from build123d import *

# Parameters (mm, degrees)
SKETCH1_W                = 21
SKETCH1_H                = 145.5
SKETCH1_W_2              = 11
SKETCH1_H_2              = 21
BOSS_EXTRUDE1_DEPTH      = 2
BOSS_EXTRUDE2_DEPTH      = 30
BOSS_EXTRUDE2_DEPTH_BACK = 2
FILLET2_R                = 2.5
SKETCH6_R                = 2
CUT_EXTRUDE1_DEPTH       = 2
BOSS_EXTRUDE5_DEPTH      = 1
BOSS_EXTRUDE6_DEPTH      = 1
SKETCH9_R                = 2
CUT_EXTRUDE2_DEPTH       = 2
FILLET3_R                = 1


with BuildPart() as part:
    # Sketch1 → Boss-Extrude1 (new body)
    with BuildSketch(Plane.XY):
        Rectangle(SKETCH1_W, SKETCH1_H)
        with Locations((0, -42.75)):
            Rectangle(SKETCH1_W_2, SKETCH1_H_2, mode=Mode.SUBTRACT)
        with Locations((0, 7.25)):
            Rectangle(SKETCH1_W_2, SKETCH1_H_2, mode=Mode.SUBTRACT)
        with Locations((0, 57.25)):
            Rectangle(SKETCH1_W_2, SKETCH1_H_2, mode=Mode.SUBTRACT)
    extrude(amount=BOSS_EXTRUDE1_DEPTH)

    # Sketch2 → Boss-Extrude2 (add, two sides: drawn at the far end of the back side and taken through both)
    with BuildSketch(Plane(origin=(0, 0, 0), x_dir=(-1, 0, 0), z_dir=(0, 0, -1)).offset(-BOSS_EXTRUDE2_DEPTH_BACK)):
        Polygon((10.5, -72.75), (16.5, -72.75), (16.5, -74.75), (-16.5, -74.75), (-16.5, -72.75), align=None)
    extrude(amount=BOSS_EXTRUDE2_DEPTH + BOSS_EXTRUDE2_DEPTH_BACK)

    # Fillet2
    # the kernel refuses this fillet: 2.5 mm, written as the material it takes off along each edge
    with BuildSketch(Plane(origin=(22.623724357, -72.75, -30), x_dir=(0, 0, 1), z_dir=(-1, 0, 0))) as fillet2_piece_1:
        with BuildLine():
            CenterArc((2.449489743, -2.5), FILLET2_R, 90, 78.463040967)
            Line((0, -2), (-0.048989795, -1.99))
            ThreePointArc((-0.048989795, -1.99), (-0.05, -1), (-0.05, 0))
            Line((-0.05, 0), (0, 0.05))
            Line((0, 0.05), (2.449489743, 0.05))
            Line((2.449489743, 0.05), (2.449489743, 0))
        make_face()
    extrude(amount=45.247448714, mode=Mode.SUBTRACT)

    # Sketch6 → Cut-Extrude1 (cut)
    with BuildSketch(Plane(origin=(0, -72.75, 0), x_dir=(1, 0, 0), z_dir=(0, 1, 0))):
        with Locations(Location((0, 24, 0), (0, 0, 270))):
            Circle(SKETCH6_R)
    extrude(amount=-CUT_EXTRUDE1_DEPTH, mode=Mode.SUBTRACT)

    # Sketch7 → Boss-Extrude5 (add, symmetric)
    with BuildSketch(Plane(origin=(7.5, 0, 0), x_dir=(0, 0, -1), z_dir=(1, 0, 0))):
        Polygon((0, -53.25), (12, -72.75), (0, -72.75), align=None)
    extrude(amount=BOSS_EXTRUDE5_DEPTH, both=True)

    # Sketch8 → Boss-Extrude6 (add, symmetric)
    with BuildSketch(Plane(origin=(-7.5, 0, 0), x_dir=(0, 0, -1), z_dir=(1, 0, 0))):
        Polygon((12, -72.75), (0, -53.25), (0, -72.75), align=None)
    extrude(amount=BOSS_EXTRUDE6_DEPTH, both=True)

    # Sketch9 → Cut-Extrude2 (cut)
    with BuildSketch(Plane.XZ.offset(74.75)):
        with Locations(Location((13, -24, 0), (0, 0, 270))):
            Circle(SKETCH9_R)
        with Locations(Location((-13, -24, 0), (0, 0, 90))):
            Circle(SKETCH9_R)
    extrude(amount=-CUT_EXTRUDE2_DEPTH, mode=Mode.SUBTRACT)

    # Fillet3
    fillet3_edges = [part.edges().sort_by_distance(p)[0] for p in [
        (-9.5, -72.75, 0),
        (10.5, -72.75, 1),
        (-10.5, -72.75, 1),
        (9.5, -72.75, 0),
        (6.5, -72.75, -6),
        (8.5, -72.75, -6),
        (0, -72.75, 0),
        (-8.5, -72.75, -6),
        (-6.5, -72.75, -6),
    ]]
    fillet(fillet3_edges, radius=FILLET3_R)


solid = part.part
The model under review builds one solid part; all positions refer to its coordinate system, in mm. A direction names the side the tool comes from. Coordinates: 2 decimals unless noted, no trailing zeros. Loops run counter-clockwise (first coordinate to the right, second up) from the corner with the lowest first, then second, coordinate; pieces in that order, holes last.
(1) Draft analysis for pull direction Z (two halves, no side actions). For faces 1 (the flat face through (8, -63, -6)), 2 (the cylindrical face through (-14.352, -73.764, -25.474)), 3 (the flat face through (0, -6, 2)), 4 (the flat face through (6.5, -66, -3)), state which applies: +Z half, -Z half, draft (parallel to the pull), parting line (faces both ways), or undercut.
Determined:
face 1: -Z half
face 2: undercut
face 3: +Z half
face 4: draft
(2) Consider section D-D, the plane x = 0. Give the boundary of the cut face in (y, z).
Determined:
outline: (-74.75, -30) arc R2.5 ccw to (-72.75, -27.55) - (-72.75, -26) - (-74.75, -26) - close; (-74.75, -22) - (-72.75, -22) - (-72.75, -1) arc R1 cw to (-71.75, 0) - (-53.25, 0) - (-53.25, 2) - (-74.75, 2) - close; (-32.25, 0) - (-3.25, 0) - (-3.25, 2) - (-32.25, 2) - close; (17.75, 0) - (46.75, 0) - (46.75, 2) - (17.75, 2) - close; (67.75, 0) - (72.75, 0) - (72.75, 2) - (67.75, 2) - close
(3) Consider section A-A, the plane x = 13. Give the boundary of the cut face in (y, z), plus the area to 3 significant figures.
Determined:
outline: (-74.75, -30) arc R2.5 ccw to (-72.75, -27.55) - (-72.75, -26) - (-74.75, -26) - close; (-74.75, -22) - (-72.75, -22) - (-72.75, 2) - (-74.75, 2) - close
area: 54.8 mm2
(4) Consider section B-B, the plane y = 56. Give the boundary of the cut face in (x, z).
Determined:
outline: (-10.5, 0) - (-5.5, 0) - (-5.5, 2) - (-10.5, 2) - close; (5.5, 0) - (10.5, 0) - (10.5, 2) - (5.5, 2) - close
(5) Consider section C-C, the plane z = -24. Give the boundary of the cut face in (x, y), plus the area to 3 significant figures.
Determined:
outline: (-16.5, -74.75) - (-15, -74.75) - (-15, -72.75) - (-16.5, -72.75) - close; (-11, -74.75) - (-2, -74.75) - (-2, -72.75) - (-11, -72.75) - close; (2, -74.75) - (11, -74.75) - (11, -72.75) - (2, -72.75) - close; (15, -74.75) - (16.5, -74.75) - (16.5, -72.75) - (15, -72.75) - close
area: 42.0 mm2
(6) Wall thickness on L1, parallel to X at y = -73.9, z = -24; L2, parallel to Y at x = 3, z = 0.5; L3, parallel to Z at x = -7, y = 66: over which ranges is each line inside the solid? List them lowest first.
Determined:
L1: x = -16.5 to -15, -11 to -2, 2 to 11, 15 to 16.5
L2: y = -74.75 to -53.25, -32.25 to -3.25, 17.75 to 46.75, 67.75 to 72.75
L3: z = 0 to 2
(7) Insertion check: P1, Ø2, axis at y = -40, z = 1.5, coming from the +X side; P2, Ø0.6, axis at y = 58, z = 1, coming from the -X side; P3, Ø5, axis at x = -7.5, z = -6, coming from the +Y side; P4, Ø1, axis at x = 12, y = -40, coming from the -Z side. Each pin has a flat end and moves straight along its axis. Give the tip position at first contact, or say it passes through.
Determined:
P1: stops at x = 10.5
P2: stops at x = -10.5
P3: stops at y = -58.94
P4: passes through
(8) Tool access review of faces 5 (the flat face through (0, -72.75, -13)), 6 (the flat face through (8.5, -66, -3)), 7 (the flat face through (-8.5, -66, -3)), 8 (the cylindrical face through (-1.2, -73.7, -25.6)): name each direction out of +Z, -Z, +X, -X, +Y, -Y from which nothing blocks a thin tool from reaching the whole face with its end or side.
Determined:
face 5: -Z, +Y
face 6: -Z, +X, +Y
face 7: -Z, -X, +Y
face 8: +Y, -Y
